Source: CAD feature listing. Evaluate the final solid. Frame: model axes, mm. Face numbers are marked on the shaded views. A direction names the side the tool comes from. Give positions to 0.01 mm unless a question says otherwise; leave off trailing zeros. Loops run counter-clockwise (first coordinate to the right, second up) from the corner with the lowest first, then second, coordinate; pieces in that order, holes last.
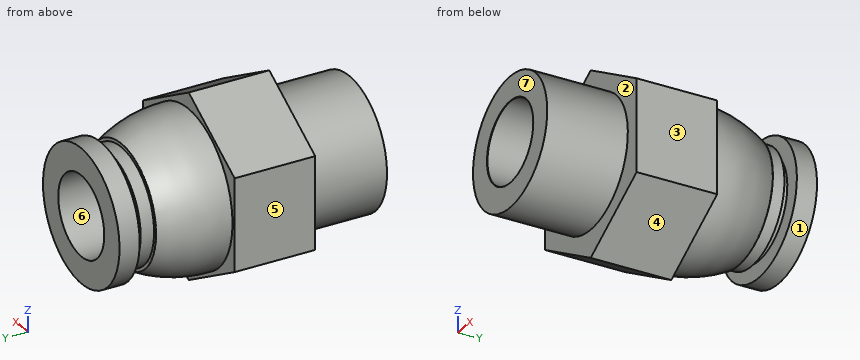
from build123d import *

# Parameters (mm, degrees)
SKETCH_1_R            = 4.85
EXTRUDE_1_DEPTH       = 6
EXTRUDE_2_DEPTH       = 6
SKETCH_3_R            = 4.5
EXTRUDE_3_DEPTH       = 5
SKETCH_4_R            = 4.25
EXTRUDE_4_DEPTH       = 1
SKETCH_5_R            = 3.75
EXTRUDE_5_DEPTH       = 0.5
SKETCH_6_R            = 5
EXTRUDE_6_DEPTH       = 1.5
F_6_0MM_1_D           = 6
F_6_0MM_1_CSINK_D     = 6.05
F_6_0MM_1_CSINK_ANGLE = 90


with BuildPart() as part:
    # 草图1 → 凸台-拉伸1 (new body)
    with BuildSketch(Plane(origin=(0, 0, 0), x_dir=(1, 0, 0), z_dir=(0, 1, 0))):
        with Locations(Location((0, 0, 0), (0, 0, 270))):
            Circle(SKETCH_1_R)
    extrude(amount=EXTRUDE_1_DEPTH)

    # 草图2 → 凸台-拉伸2 (add)
    with BuildSketch(Plane(origin=(0, 6, 0), x_dir=(1, 0, 0), z_dir=(0, 1, 0))):
        Polygon((6, 3.464101615), (0, 6.92820323), (-6, 3.464101615), (-6, -3.464101615), (0, -6.92820323), (6, -3.464101615), align=None)
    extrude(amount=EXTRUDE_2_DEPTH)

    # 草图3 → 凸台-拉伸3 (add)
    with BuildSketch(Plane(origin=(0, 12, 0), x_dir=(1, 0, 0), z_dir=(0, 1, 0))):
        with Locations(Location((0, 0, 0), (0, 0, 270))):
            Circle(SKETCH_3_R)
    extrude(amount=EXTRUDE_3_DEPTH)

    # 草图4 → 凸台-拉伸4 (add)
    with BuildSketch(Plane(origin=(0, 17, 0), x_dir=(1, 0, 0), z_dir=(0, 1, 0))):
        with Locations(Location((0, 0, 0), (0, 0, 270))):
            Circle(SKETCH_4_R)
    extrude(amount=EXTRUDE_4_DEPTH)

    # 草图5 → 凸台-拉伸5 (add)
    with BuildSketch(Plane(origin=(0, 18, 0), x_dir=(1, 0, 0), z_dir=(0, 1, 0))):
        with Locations(Location((0, 0, 0), (0, 0, 270))):
            Circle(SKETCH_5_R)
    extrude(amount=EXTRUDE_5_DEPTH)

    # 草图6 → 凸台-拉伸6 (add)
    with BuildSketch(Plane(origin=(0, 18.5, 0), x_dir=(1, 0, 0), z_dir=(0, 1, 0))):
        with Locations(Location((0, 0, 0), (0, 0, 270))):
            Circle(SKETCH_6_R)
    extrude(amount=EXTRUDE_6_DEPTH)

    # 草图7 → 旋转1 (revolve)
    with BuildSketch(Plane.XY, mode=Mode.PRIVATE) as revolve_1_sk:
        with BuildLine():
            Line((-5.71614298, 12), (-4.5, 12))
            Line((-4.5, 12), (-4.5, 16.986349243))
            add(Edge.make_bspline(
                [(-4.5, 16.986349243), (-5.756767144, 14.677598977), (-5.71614298, 12)],
                knots=[0, 0, 0, 1, 1, 1], degree=2))
        make_face()
    revolve(revolve_1_sk.sketch.rotate(Axis((0, 12, 0), (0, 1, 0)), 180), axis=Axis((0, 12, 0), (0, 1, 0)))

    # Ø6.0mm 暗销孔1 (through all)
    with Locations(Plane(origin=(0, 0, 0), x_dir=(-1, 0, 0), z_dir=(0, -1, 0))):
        with Locations((0, 0)):
            CounterSinkHole(F_6_0MM_1_D / 2, F_6_0MM_1_CSINK_D / 2, counter_sink_angle=F_6_0MM_1_CSINK_ANGLE)


solid = part.part
1) Ray query, probe 1 along Y at (x, z) = (1, 4.25); probe 2 along Y at (x, z) = (3.5, -2); probe 3 along Z at (x, y) = (1, 10). Return the intervals inside material, ascending.
Checks:
probe 1: y = 0 to 17, 18.5 to 20
probe 2: y = 0 to 18, 18.5 to 20
probe 3: z = -6.35 to -2.83, 2.83 to 6.35
2) Pull-direction query (X, two-part tool) for the marked faces 4, 5, 6 and 7; classes: released by +X, released by -X, zero draft, split by the parting line, or undercut.
Checks:
face 4: released by +X
face 5: released by -X
face 6: undercut
face 7: zero draft
3) Contact query for a flat-ended pin moving along its axis: P1, Ø1.5, axis at x = -2.5, y = 18, coming from the -Z side. Output: stop coordinate, or through.
Checks:
P1: stops at z = -4.61
4) Cut plane A-A (y = 6.25). Return loops of the section in (x, z).
Checks:
outline: (-6, -3.46) - (0, -6.93) - (6, -3.46) - (6, 3.46) - (0, 6.93) - (-6, 3.46) - close; hole circle Ø6 at (0, 0)
5) Reachability of the marked faces 1, 2 and 3 from +Z, -Z, +X, -X, +Y, -Y: full face, straight path, thin tool, end or side. Return the list, or none.
Checks:
face 1: +Y
face 2: -Y
face 3: +Z, -Z, +X, +Y, -Y
